from build123d import *

# Parameters (mm, degrees)
CROQUIS1_R              = 3.8
CROQUIS1_R_2            = 2.8
SALIENTE_EXTRUIR1_DEPTH = 19.5
CROQUIS1_4_R            = 2.8
SALIENTE_EXTRUIR2_DEPTH = 8.5
REDONDEO1_R             = 1
REDONDEO2_R             = 0.5


with BuildPart() as part:
    # Croquis1 → Saliente-Extruir1 (new body)
    # profile 1 of 2: a face of its own
    with BuildSketch(Plane.YZ):
        with Locations(Location((0, 0, 0), (0, 0, 270))):
            Circle(CROQUIS1_R)
        Circle(CROQUIS1_R_2, mode=Mode.SUBTRACT)
    # profile 2 of 2: a face of its own
    with BuildSketch(Plane.YZ):
        Circle(CROQUIS1_R_2)
    extrude(amount=SALIENTE_EXTRUIR1_DEPTH)

    # Croquis1<4> → Saliente-Extruir2 (add)
    with BuildSketch(Plane.YZ):
        with Locations(Location((0, 0, 0), (0, 0, 270))):
            Circle(CROQUIS1_4_R)
    extrude(amount=-SALIENTE_EXTRUIR2_DEPTH)

    # Redondeo1
    redondeo1_edges = [part.edges().sort_by_distance(p)[0] for p in [
        (19.5, 0, 3.8),
        (0, 0, 2.8),
    ]]
    fillet(redondeo1_edges, radius=REDONDEO1_R - 0.0001)  # a hair under: the kernel refuses the full size

    # Redondeo2
    redondeo2_edges = [part.edges().sort_by_distance(p)[0] for p in [
        (-8.5, 0, 2.8),
    ]]
    fillet(redondeo2_edges, radius=REDONDEO2_R)


solid = part.part
Build history of the part. All positions in model axes, mm. A direction names the side the tool comes from. Coordinates: 2 decimals unless noted, no trailing zeros. Order: outer loops, then holes, each group sorted by start corner. A loop starts at its lowest first (then second) coordinate and runs counter-clockwise, first axis right, second up. Notation, with made-up numbers: (37, 6) - (78, 6) arc R14 ccw to (78, 16) - close; hole circle Ø3 at (42, 10). An arc over 180 degrees is marked (long way). Put each result on its own line as item: value.
1. Probe line 1 along Y through (x, z) = (-1.75, 1); line 2 along X through (y, z) = (2.5, 2); line 3 along Z through (x, y) = (1.25, 1). List the from-to ranges inside material, lowest first. Write a range as [from, to].
Answer sheet:
line 1: y = [-2.62, 2.62]
line 2: x = [-0.2, 19.42]
line 3: z = [-3.67, 3.67]
2. Drop flat-ended pins along their axis: P1, Ø1.5, axis at y = 3, z = 0.5, coming from the +X side; P2, Ø2, axis at x = 15.5, y = -1.5, coming from the +Z side; P3, Ø1.5, axis at x = 7, z = 2, coming from the -Y side; P4, Ø1, axis at x = 2, z = 1.5, coming from the -Y side. Give the stop position or say it passes through.
Answer sheet:
P1: stops at x = 19.5
P2: stops at z = 3.77
P3: stops at y = -3.59
P4: stops at y = -3.67
3. Tool access for faces 1 (the face through (-4.5, 0.1, 2.8)), 2 (the face through (9.12, -1.46, -3.51)): list every direction of +Z, -Z, +X, -X, +Y, -Y with a clear straight run to the whole face (end or side of a thin tool).
Answer sheet:
face 1: -X
face 2: +X, -X
4. Saw through at C-C (x = 5.5). Write the cut outline in (y, z), and give its area (3 significant figures).
Answer sheet:
outline: circle Ø7.6 at (0, 0)
area: 45.4 mm^2
